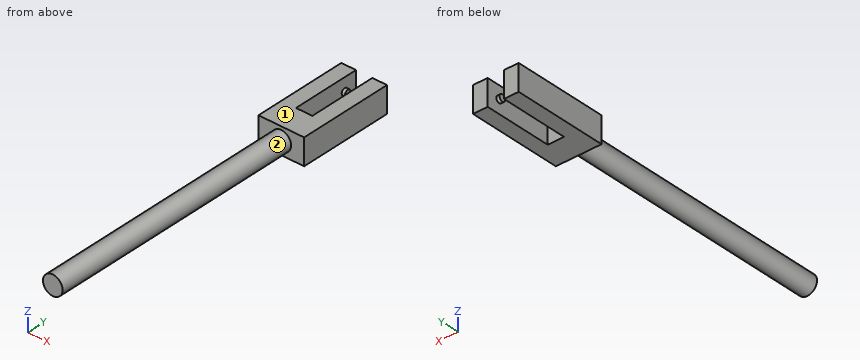
from build123d import *

# Parameters (mm, degrees)
F0_R     = 4.7625
F1_DEPTH = 127
F2_W     = 22.225
F2_H     = 12.7
F3_DEPTH = 46.0375
F4_W     = 7.9375
F4_H     = 12.7
F5_DEPTH = 33.3375
F6_R     = 1.5875
F7_DEPTH = 1.59258


with BuildPart() as f1:
    # F0 (on Front) → F1 (new body)
    with BuildSketch(Plane.XZ):
        Circle(F0_R)
    extrude(amount=F1_DEPTH)

    # F2 (on face) → F3 (join)
    with BuildSketch(Plane(origin=(0, 0, 0), x_dir=(-1, 0, 0), z_dir=(0, 1, 0))):
        Rectangle(F2_W, F2_H)
    extrude(amount=F3_DEPTH)

    # F4 (on face) → F5 (cut)
    with BuildSketch(Plane(origin=(0, 46.0375, 0), x_dir=(-1, 0, 0), z_dir=(0, 1, 0))):
        Rectangle(F4_W, F4_H)
    extrude(amount=-F5_DEPTH, mode=Mode.SUBTRACT)

    # F6 (on face) → F7 (join)
    with BuildSketch(Plane.YZ.offset(-3.96875)):
        with Locations((39.6875, 0)):
            Circle(F6_R)
    extrude(amount=F7_DEPTH)

    # F8: F1 across plane


with BuildPart() as f1_1:
    add(f1.part)
    add(f1.part.mirror(Plane.YZ))


solid = f1_1.part
Read the model definition and answer for the solid it produces. Units are mm, in the model's axes. Face numbers are marked on the shaded views. A direction names the side the tool comes from. Give positions to 0.01 mm unless a question says otherwise; leave off trailing zeros. Loops run counter-clockwise (first coordinate to the right, second up) from the corner with the lowest first, then second, coordinate; pieces in that order, holes last. Notation, with made-up numbers: (81, 86.5) -> (117, 86.5) arc R25 cw to (117, 122.5) -> close; hole circle Ø11 at (-3.75, 27.5). An arc over 180 degrees is marked (long way). Use a Markdown table: item, result.
Q1. Section B-B, the plane x = 0 is taken. Determine the outline of the cut face in (y, z).
Solved:
| item | result |
|---|---|
| outline | (-127, -4.76) -> (0, -4.76) -> (0, -6.35) -> (12.7, -6.35) -> (12.7, 6.35) -> (0, 6.35) -> (0, 4.76) -> (-127, 4.76) -> close |
Q2. Section C-C, the plane y = -10 is taken. Determine the outline of the cut face in (x, z) (1 decimal).
Solved:
| item | result |
|---|---|
| outline | circle Ø9.5 at (0, 0) |
Q3. Find the intervals of material crossed by line 1 along X through (y, z) = (21.5, 4); line 2 along Y through (x, z) = (3, -4.5); line 3 along Y through (x, z) = (-9.5, 2.75), in increasing order.
Solved:
| item | result |
|---|---|
| line 1 | x = -11.11 to -3.97, 3.97 to 11.11 |
| line 2 | y = 0 to 12.7 |
| line 3 | y = 0 to 46.04 |
Q4. Section A-A, the plane z = 0 is taken. Determine the outline of the cut face in (x, y) (1 decimal).
Solved:
| item | result |
|---|---|
| outline | (-11.1, 0) -> (-4.8, 0) -> (-4.8, -127) -> (4.8, -127) -> (4.8, 0) -> (11.1, 0) -> (11.1, 46) -> (4, 46) -> (4, 41.3) -> (2.4, 41.3) -> (2.4, 38.1) -> (4, 38.1) -> (4, 12.7) -> (-4, 12.7) -> (-4, 38.1) -> (-2.4, 38.1) -> (-2.4, 41.3) -> (-4, 41.3) -> (-4, 46) -> (-11.1, 46) -> close |
Q5. A tool of negligible diameter and unlimited length cuts with its end or side. For the marked faces 1 and 2, from which of +Z, -Z, +X, -X, +Y, -Y can it reach the whole face along a straight path? Write none if from no direction.
Solved:
| item | result |
|---|---|
| face 1 | +Z, +X, -X, +Y, -Y |
| face 2 | -Y |
Q6. Section D-D, the plane x = 8 is taken. Determine the outline of the cut face in (y, z), then the cut area to 3 significant figures.
Solved:
| item | result |
|---|---|
| outline | (0, -6.35) -> (46.04, -6.35) -> (46.04, 6.35) -> (0, 6.35) -> close |
| area | 585 mm^2 |
Q7. Each of these flat-tipped pins is pushed along its axis until it touches: pin 1 (5 mm diameter, centred on y = -6, z = 1.5, fed in from -X); pin 2 (2 mm diameter, centred on x = 0.5, z = 0, fed in from +Y); pin 3 (2 mm diameter, centred on x = 1.5, y = -101.5, fed in from +Z). Where does it stop, or does it pass through?
Solved:
| item | result |
|---|---|
| pin 1 | stops at x = -4.76 |
| pin 2 | stops at y = 12.7 |
| pin 3 | stops at z = 4.74 |
